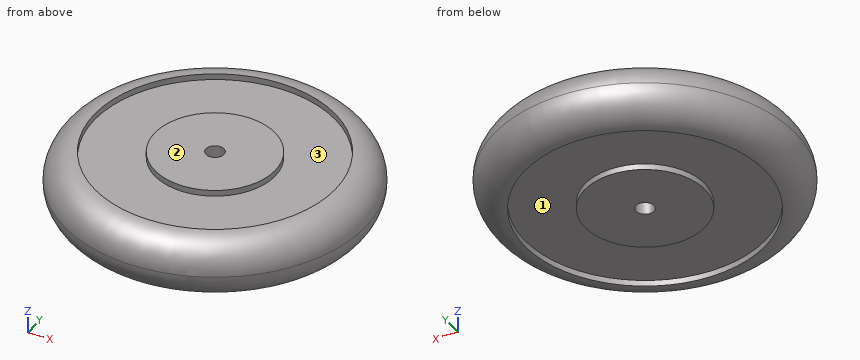
from build123d import *

# Parameters (mm, degrees)
F0_R     = 25
F0_R_2   = 20
F1_DEPTH = 5
F0_R_3   = 10
F2_DEPTH = 4
F3_R     = 4.99999
F5_D     = 3
F5_DEPTH = 250
F5_TIP   = 0.9012909285


# Not quite as in the source:
# - a fillet or chamfer is up to 0.001 mm smaller than in the source, because OpenCascade refuses the exact size


with BuildPart() as f1:
    # F0 (on Top) → F1 (new body, symmetric)
    with BuildSketch(Plane.XY):
        Circle(F0_R)
        Circle(F0_R_2, mode=Mode.SUBTRACT)
    extrude(amount=F1_DEPTH, both=True)



with BuildPart() as f1b:
    # F0 (on Top) → F1, piece 2 (new body, symmetric)
    with BuildSketch(Plane.XY):
        Circle(F0_R_3)
    extrude(amount=F1_DEPTH, both=True)


with BuildPart() as f1_1:
    add(f1.part)

    add(f1b.part)  # F2 merges F1b
    # F0 (on Top) → F2 (join, symmetric)
    with BuildSketch(Plane.XY):
        Circle(F0_R_2)
        Circle(F0_R_3, mode=Mode.SUBTRACT)
    extrude(amount=F2_DEPTH, both=True)

    # F3 (radius 5 in the source; OpenCascade refuses exactly that, so slightly less here)
    f3_edges = [f1_1.edges().sort_by_distance(p)[0] for p in [
        (-25, 0, 5),
        (-25, 0, -5),
    ]]
    fillet(f3_edges, radius=F3_R)

    # F5
    with Locations(Plane(origin=(0, 0, -5), x_dir=(1, 0, 0), z_dir=(0, 0, -1))):
        with Locations((0, 0)):
            Hole(F5_D / 2, depth=F5_DEPTH)
            with Locations((0, 0, -(F5_DEPTH + F5_TIP / 2))):  # 118° drill point
                Cone(0, F5_D / 2, F5_TIP, mode=Mode.SUBTRACT)


solid = f1_1.part
The listing builds one solid part. Answer for the finished solid, in the listing's coordinates (mm). Face numbers are marked on the shaded views. Coordinates: 2 decimals unless noted, no trailing zeros. Loops run counter-clockwise (first coordinate to the right, second up) from the corner with the lowest first, then second, coordinate; pieces in that order, holes last.
1) Flat-ended cylindrical pins translate along their axes: pin 1 Ø12 at (x, y) = (-15.5, 6) entering from -Z; pin 2 Ø4 at (y, z) = (-17, -3.5) entering from +X; pin 3 Ø4 at (y, z) = (9.5, -2.5) entering from -X; pin 4 Ø2 at (y, z) = (1.5, 2.5) entering from -X. Find the tip coordinate at first contact, or state that the pin passes through.
2) Find the intervals of material crossed by L1, parallel to Z at x = -14, y = -13; L2, parallel to Y at x = 0, z = 4.35; L3, parallel to Z at x = 16, y = -12.5, in increasing order.
3) Find section C-C on z = -1.25. Write down the section's boundary in (x, y).
4) Determine the mould class of the marked faces 1, 2 and 3 for opening direction X: pulls with the +X half, pulls with the -X half, needs draft (parallel to the pull), parting line crosses it, or undercut.
5) Find section D-D on z = 2.75. Write down the section's boundary in (x, y), then the cut area to 3 significant figures.
Values:
1. pin 1: stops at z = -5
1. pin 2: stops at x = 18.98
1. pin 3: stops at x = -23.54
1. pin 4: stops at x = -24.73
2. L1: z = -4 to 4
2. L2: y = -22.47 to -20, -10 to -1.5, 1.5 to 10, 20 to 22.47
2. L3: z = -4.99 to 4.99
3. outline: circle Ø49.68 at (0, 0); hole circle Ø3 at (0, 0)
4. face 1: undercut
4. face 2: needs draft
4. face 3: undercut
5. outline: circle Ø48.35 at (0, 0); hole circle Ø3 at (0, 0)
5. area: 1,830 mm2
